```python
from build123d import *

# Parameters (mm, degrees)
SKETCH1_W           = 156
SKETCH1_H           = 144
BOSS_EXTRUDE1_DEPTH = 2
SKETCH2_R           = 1.575
CUT_EXTRUDE1_DEPTH  = 5
SKETCH3_R           = 4.85
CUT_EXTRUDE2_DEPTH  = 50
SKETCH4_W           = 156
SKETCH4_H           = 144
SKETCH4_W_2         = 155.6
SKETCH4_H_2         = 143.6
CUT_EXTRUDE3_DEPTH  = 50
FILLET1_R           = 3
FILLET2_R           = 2
SKETCH5_R           = 9
SKETCH5_R_2         = 4.85
BOSS_EXTRUDE2_DEPTH = 0.5
SKETCH6_R           = 9
SKETCH6_R_2         = 5.65
BOSS_EXTRUDE3_DEPTH = 1
SKETCH7_W           = 2.2
SKETCH7_H           = 2.3
CUT_EXTRUDE4_DEPTH  = 2.5
CUT_EXTRUDE5_DEPTH  = 10


with BuildPart() as part:
    # Sketch1 → Boss-Extrude1 (new body)
    with BuildSketch(Plane(origin=(0, 0, 0), x_dir=(1, 0, 0), z_dir=(0, 1, 0))):
        with Locations((78, -72)):
            Rectangle(SKETCH1_W, SKETCH1_H)
    extrude(amount=BOSS_EXTRUDE1_DEPTH)

    # Sketch2 → Cut-Extrude1 (cut)
    with BuildSketch(Plane(origin=(0, 2, 0), x_dir=(1, 0, 0), z_dir=(0, 1, 0))):
        with Locations((3.5, -3.5)):
            Circle(SKETCH2_R)
        with Locations((152.5, -3.5)):
            Circle(SKETCH2_R)
        with Locations((152.5, -140.5)):
            Circle(SKETCH2_R)
        with Locations((3.5, -140.5)):
            Circle(SKETCH2_R)
    extrude(amount=-CUT_EXTRUDE1_DEPTH, mode=Mode.SUBTRACT)

    # Sketch3 → Cut-Extrude2 (cut)
    with BuildSketch(Plane(origin=(0, 2, 0), x_dir=(1, 0, 0), z_dir=(0, 1, 0))):
        with Locations((11, -31)):
            Circle(SKETCH3_R)
        with BuildLine():
            Line((36, -26), (101, -26))
            ThreePointArc((101, -26), (105, -30), (101, -34))
            Line((101, -34), (36, -34))
            ThreePointArc((36, -34), (32, -30), (36, -26))
        make_face()
        with BuildLine():
            Line((36, -41), (101, -41))
            ThreePointArc((101, -41), (105, -45), (101, -49))
            Line((101, -49), (36, -49))
            ThreePointArc((36, -49), (32, -45), (36, -41))
        make_face()
        with BuildLine():
            Line((36, -56), (101, -56))
            ThreePointArc((101, -56), (105, -60), (101, -64))
            Line((101, -64), (36, -64))
            ThreePointArc((36, -64), (32, -60), (36, -56))
        make_face()
        with BuildLine():
            Line((36, -71), (101, -71))
            ThreePointArc((101, -71), (105, -75), (101, -79))
            Line((101, -79), (36, -79))
            ThreePointArc((36, -79), (32, -75), (36, -71))
        make_face()
        with BuildLine():
            Line((36, -86), (101, -86))
            ThreePointArc((101, -86), (105, -90), (101, -94))
            Line((101, -94), (36, -94))
            ThreePointArc((36, -94), (32, -90), (36, -86))
        make_face()
    extrude(amount=-CUT_EXTRUDE2_DEPTH, mode=Mode.SUBTRACT)

    # Sketch4 → Cut-Extrude3 (cut)
    with BuildSketch(Plane(origin=(0, 2, 0), x_dir=(1, 0, 0), z_dir=(0, 1, 0))):
        with Locations((78, -72)):
            Rectangle(SKETCH4_W, SKETCH4_H)
        with Locations((78, -72)):
            Rectangle(SKETCH4_W_2, SKETCH4_H_2, mode=Mode.SUBTRACT)
    extrude(amount=-CUT_EXTRUDE3_DEPTH, mode=Mode.SUBTRACT)

    # Fillet1
    fillet1_edges = [part.edges().sort_by_distance(p)[0] for p in [
        (0.2, 1, 0.2),
        (155.8, 1, 0.2),
        (0.2, 1, 143.8),
    ]]
    fillet(fillet1_edges, radius=FILLET1_R)

    # Fillet2
    fillet2_edges = [part.edges().sort_by_distance(p)[0] for p in [
        (155.8, 1, 143.8),
    ]]
    fillet(fillet2_edges, radius=FILLET2_R)

    # Sketch5 → Boss-Extrude2 (add)
    with BuildSketch(Plane.XZ):
        with Locations((11, 31)):
            Circle(SKETCH5_R)
        with Locations((11, 31)):
            Circle(SKETCH5_R_2, mode=Mode.SUBTRACT)
    extrude(amount=BOSS_EXTRUDE2_DEPTH)

    # Sketch6 → Boss-Extrude3 (add)
    with BuildSketch(Plane.XZ.offset(0.5)):
        with Locations((11, 31)):
            Circle(SKETCH6_R)
        with Locations((11, 31)):
            Circle(SKETCH6_R_2, mode=Mode.SUBTRACT)
    extrude(amount=BOSS_EXTRUDE3_DEPTH)

    # Sketch7 → Cut-Extrude4 (cut)
    with BuildSketch(Plane.XZ.offset(1.5)):
        with Locations((11, 25.35)):
            Rectangle(SKETCH7_W, SKETCH7_H)
    extrude(amount=-CUT_EXTRUDE4_DEPTH, mode=Mode.SUBTRACT)

    # Sketch8 → Cut-Extrude5 (cut)
    with BuildSketch(Plane(origin=(0, 2, 0), x_dir=(1, 0, 0), z_dir=(0, 1, 0))):
        with BuildLine():
            Line((3.2, -143.8), (153.8, -143.8))
            ThreePointArc((153.8, -143.8), (155.214213562, -143.214213562), (155.8, -141.8))
            Line((155.8, -141.8), (155.8, -3.2))
            ThreePointArc((155.8, -3.2), (154.921320344, -1.078679656), (152.8, -0.2))
            Line((152.8, -0.2), (3.2, -0.2))
            ThreePointArc((3.2, -0.2), (1.078679656, -1.078679656), (0.2, -3.2))
            Line((0.2, -3.2), (0.2, -140.8))
            ThreePointArc((0.2, -140.8), (1.078679656, -142.921320344), (3.2, -143.8))
        make_face()
        with BuildLine():
            Line((3.2, -143.6), (153.8, -143.6))
            ThreePointArc((153.8, -143.6), (155.072792206, -143.072792206), (155.6, -141.8))
            Line((155.6, -141.8), (155.6, -3.2))
            ThreePointArc((155.6, -3.2), (154.779898987, -1.220101013), (152.8, -0.4))
            Line((152.8, -0.4), (3.2, -0.4))
            ThreePointArc((3.2, -0.4), (1.220101013, -1.220101013), (0.4, -3.2))
            Line((0.4, -3.2), (0.4, -140.8))
            ThreePointArc((0.4, -140.8), (1.220101013, -142.779898987), (3.2, -143.6))
        make_face(mode=Mode.SUBTRACT)
    extrude(amount=-CUT_EXTRUDE5_DEPTH, mode=Mode.SUBTRACT)


solid = part.part
```
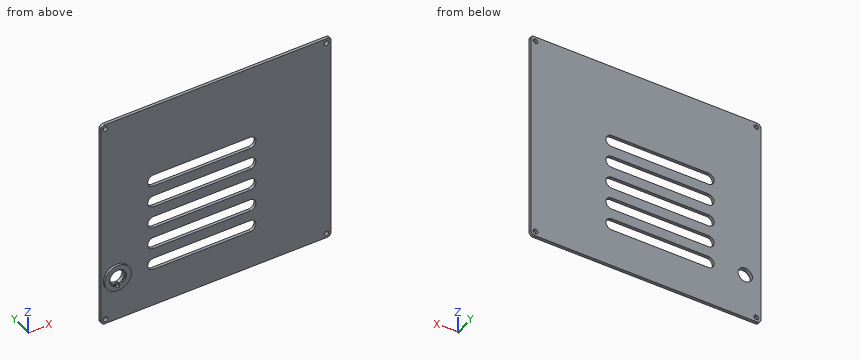
CAD build for the part. Positions are in the model's coordinates, mm. Round coordinates to 2 decimals unless told otherwise and drop trailing zeros. Order: outer loops, then holes, each group sorted by start corner. A loop starts at its lowest first (then second) coordinate and runs counter-clockwise, first axis right, second up. Notation, with made-up numbers: (-2, -5.5) - (56, -5.5) arc R25 cw to (56, 28.5) - close; hole circle Ø6 at (36.5, 67.5). An arc over 180 degrees is marked (long way). Use CSV: the item, a comma, the result in double quotes. Start each with the question number.
1) Saw through at B-B (z = 60). List the corners of the cut face in (x, y).
2) Saw through at A-A (x = 56). List the corners of the cut face in (y, z), and give its area (3 significant figures).
3) Saw through at C-C (z = 31). List the corners of the cut face in (x, y), and give its area (3 significant figures).
4) Wall check: L1, parallel to Z at x = 57, y = 0.85; L2, parallel to X at y = 0.65, z = 140.5 (3 decimals); L3, parallel to Z at x = 152.5, y = 1.4 (3 decimals). Give the ranges that are in metal, low to high. Write a range as [from, to].
5) Saw through at D-D (x = 130.5). List the corners of the cut face in (y, z).
6) Pin check, flat tips, straight feed: pin 1 Ø2.5 at (x, z) = (152.5, 140.5) entering from -Y; pin 2 Ø0.6 at (y, z) = (-1, 25) entering from +X. Stop position of each tip, or through.
Values follow:
1,outline,"(0.4, 0) - (32, 0) - (32, 2) - (0.4, 2) - close; (105, 0) - (155.6, 0) - (155.6, 2) - (105, 2) - close"
2,outline,"(0, 0.4) - (2, 0.4) - (2, 26) - (0, 26) - close; (0, 34) - (2, 34) - (2, 41) - (0, 41) - close; (0, 49) - (2, 49) - (2, 56) - (0, 56) - close; (0, 64) - (2, 64) - (2, 71) - (0, 71) - close; (0, 79) - (2, 79) - (2, 86) - (0, 86) - close; (0, 94) - (2, 94) - (2, 143.6) - (0, 143.6) - close"
2,area,"206 mm2"
3,outline,"(0.4, 0) - (2, 0) - (2, -1.5) - (5.35, -1.5) - (5.35, -0.5) - (6.15, -0.5) - (6.15, 2) - (0.4, 2) - close; (15.85, -0.5) - (16.65, -0.5) - (16.65, -1.5) - (20, -1.5) - (20, 0) - (32.13, 0) - (32.13, 2) - (15.85, 2) - close; (104.87, 0) - (155.6, 0) - (155.6, 2) - (104.87, 2) - close"
3,area,"156 mm2"
4,L1,"z = [0.4, 26], [34, 41], [49, 56], [64, 71], [79, 86], [94, 143.6]"
4,L2,"x = [0.4, 1.925], [5.075, 150.925], [154.075, 155.6]"
4,L3,"z = [0.4, 1.925], [5.075, 138.925], [142.075, 143.6]"
5,outline,"(0, 0.4) - (2, 0.4) - (2, 143.6) - (0, 143.6) - close"
6,pin 1,"passes through"
6,pin 2,"stops at x = 17.96"
